Could you check a few things on this drawing? It's one solid part, dimensions in mm from its lowest x, y, z. A direction names the side the tool comes from. Round coordinates to 2 decimals unless told otherwise and drop trailing zeros. Write each loop counter-clockwise with the first axis right and the second up, starting at its lowest first coordinate (ties: lowest second). Pieces come first, ordered by that corner, then holes. Notation, with made-up numbers: (55.5, 84.25) -> (99.5, 84.25) arc R16 ccw to (99.5, 104.25) -> close; hole circle Ø5 at (66, -37.75). An arc over 180 degrees is marked (long way). Return JSON: item names as keys, results as strings.
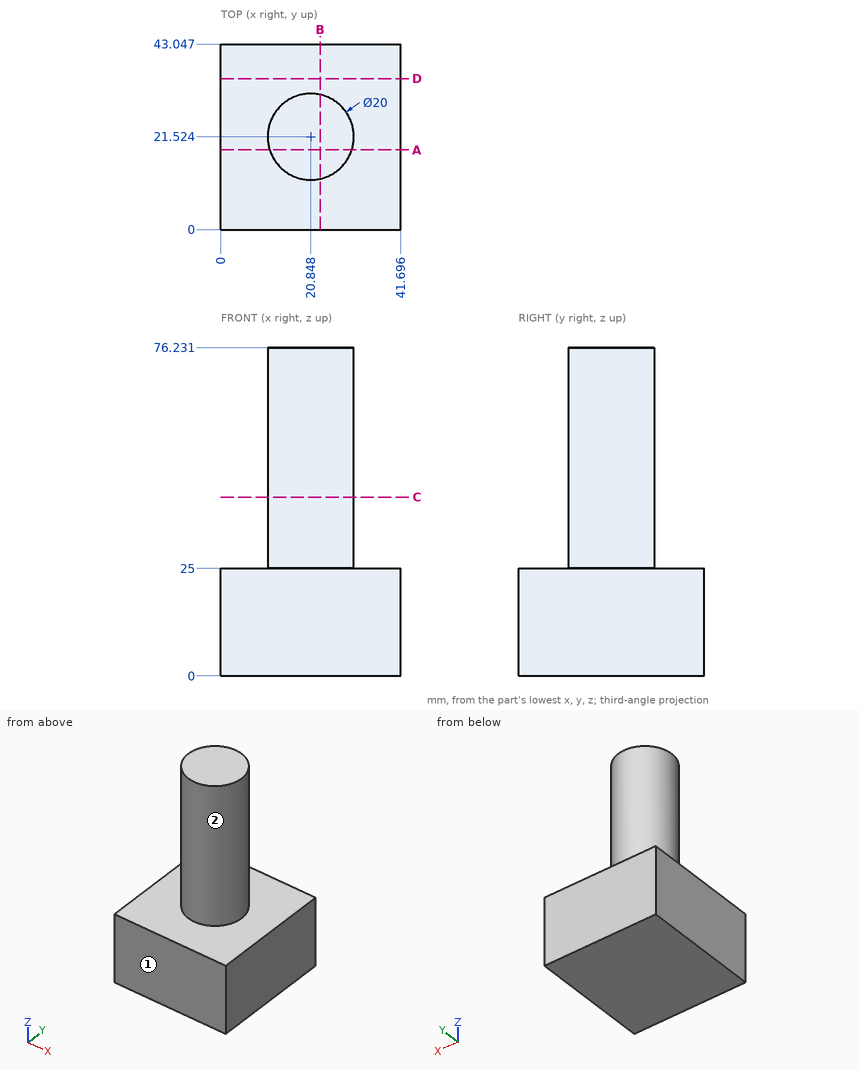
1) For the marked faces 1 and 2, which set-ups out of +Z, -Z, +X, -X, +Y, -Y let a thin tool reach every point of the face, with its end or its side?
Return value:
{"face 1": "+Z, -Z, +X, -X, -Y", "face 2": "+Z"}
2) I want a section at C-C, the plane z = 41.5. Please give me the cut outline in (x, y), and give its area (3 significant figures).
Return value:
{"outline": "circle Ø20 at (20.85, 21.52)", "area": "314 mm²"}
3) I want a section at A-A, the plane y = 18.5. Please give me the cut outline in (x, z), and give its area (3 significant figures).
Return value:
{"outline": "(0, 0) -> (41.7, 0) -> (41.7, 25) -> (30.38, 25) -> (30.38, 76.23) -> (11.32, 76.23) -> (11.32, 25) -> (0, 25) -> close", "area": "2,020 mm²"}
4) If I drill on probe 1 along Z at (x, y) = (31.5, 28.5); probe 2 along X at (y, z) = (22, 41); probe 3 along Y at (x, z) = (17, 73.5) (1 decimal), over which ranges is the centre line in solid material (lowest first)? Write a range as [from, to].
Return value:
{"probe 1": "[0, 25]", "probe 2": "[10.86, 30.84]", "probe 3": "[12.3, 30.8]"}
5) I want a section at D-D, the plane y = 35. Please give me the cut outline in (x, z), and give its area (3 significant figures).
Return value:
{"outline": "(0, 0) -> (41.7, 0) -> (41.7, 25) -> (0, 25) -> close", "area": "1,040 mm²"}
6) Will these pins go through, and if not, where does the flat tip stop? pin 1 Ø2 at (y, z) = (26.5, 56.5) entering from -X; pin 2 Ø8 at (x, y) = (25.5, 12.5) entering from +Z; pin 3 Ø2 at (y, z) = (14.5, 31) entering from +X; pin 4 Ø4 at (y, z) = (32.5, 62.5) entering from -X.
Return value:
{"pin 1": "x = 11.67", "pin 2": "z = 76.23", "pin 3": "x = 28.83", "pin 4": "x = 16.44"}
7) I want a section at B-B, the plane x = 23. Please give me the cut outline in (y, z), and give its area (3 significant figures).
Return value:
{"outline": "(0, 0) -> (43.05, 0) -> (43.05, 25) -> (31.29, 25) -> (31.29, 76.23) -> (11.76, 76.23) -> (11.76, 25) -> (0, 25) -> close", "area": "2,080 mm²"}
